Check sheet for the drawn part. Datum: minimum x, y, z corner. Units: mm. A direction names the side the tool comes from. Coordinates: 2 decimals unless noted, no trailing zeros. Loops run counter-clockwise (first coordinate to the right, second up) from the corner with the lowest first, then second, coordinate; pieces in that order, holes last.
Q1. Sectioned sample at B-B (x = 32). Enter the section's corners in (y, z) (1 decimal).
Q2. Material ranges on probe 1 along X at (y, z) = (11, 32); probe 2 along Z at (x, y) = (6.5, 25.5) (1 decimal), recorded low to high.
Q3. Access from +Z, -Z, +X, -X, +Y, -Y to the whole of each face (thin tool, end or side, straight path). Record for the marked faces 1 and 2.
Q4. Go/stop test with flat-tipped pins: P1, Ø5, axis at x = 8.5, z = 5, coming from the -Y side; P2, Ø12.5, axis at y = 11, z = 28, coming from the +X side; P3, Ø5, axis at y = 23, z = 9.5, coming from the +X side; P4, Ø7.5, axis at x = 22, y = 12.5, coming from the +Z side. Record where each tip stops, or that it passes through.
Q5. Sectioned sample at A-A (y = 24). Enter the section's corners in (x, z) (1 decimal).
Q6. Sectioned sample at C-C (z = 34.5). Enter the section's corners in (x, y) (1 decimal).
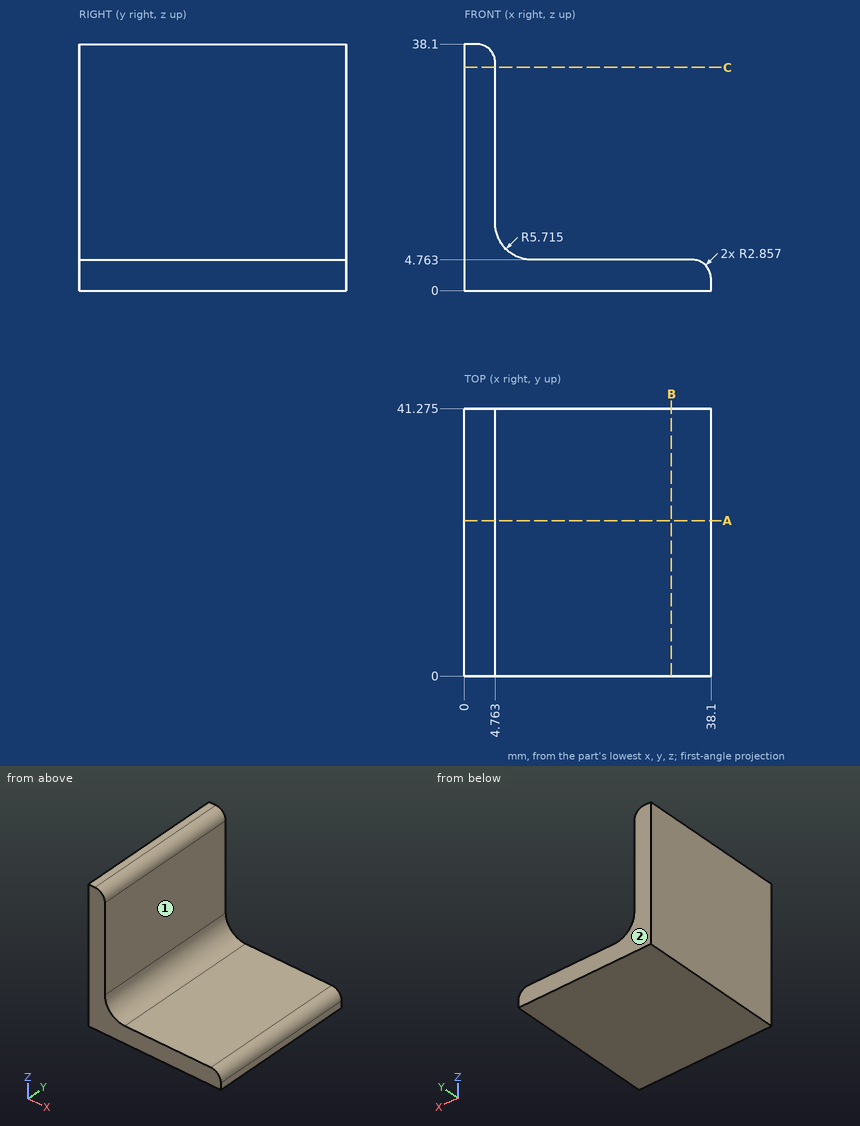
Geometry check:
1. outline: (0, 0) - (41.3, 0) - (41.3, 4.8) - (0, 4.8) - close
2. probe 1: x = 0 to 4.76
2. probe 2: z = 0 to 6.4
3. face 1: +Z, +X, +Y, -Y
3. face 2: +Z, -Z, +X, -X, +Y
4. P1: stops at y = 0
4. P2: stops at x = 4.76
4. P3: stops at x = 5.94
4. P4: stops at z = 4.76
5. outline: (0, 0) - (38.1, 0) - (38.1, 1.9) arc R2.9 ccw to (35.2, 4.8) - (10.5, 4.8) arc R5.7 cw to (4.8, 10.5) - (4.8, 35.2) arc R2.9 ccw to (1.9, 38.1) - (0, 38.1) - close
6. outline: (0, 0) - (4.8, 0) - (4.8, 41.3) - (0, 41.3) - close
